Could you check a few things on this drawing? It's one solid part, dimensions in mm from its lowest x, y, z. A direction names the side the tool comes from. Round coordinates to 2 decimals unless told otherwise and drop trailing zeros. Order: outer loops, then holes, each group sorted by start corner. A loop starts at its lowest first (then second) coordinate and runs counter-clockwise, first axis right, second up. Notation, with made-up numbers: (51.5, 49) -> (94.5, 49) arc R24 ccw to (94.5, 81) -> close; hole circle Ø11 at (32.25, -3). An arc over 180 degrees is marked (long way). Use a Markdown table: item, result. Add a question column.
(1) I want a section at C-C, the plane x = 40. Please give me the cut outline in (y, z), then the cut area to 3 significant figures.
(2) I want a section at D-D, the plane y = 83.5. Please give me the cut outline in (x, z), then the cut area to 3 significant figures.
(3) I want a section at B-B, the plane y = 11. Please give me the cut outline in (x, z), then the cut area to 3 significant figures.
(4) I'm going to push flat-ended pins straight in: P1, Ø15, axis at y = 55, z = 23, coming from the -X side; P2, Ø1.5, axis at x = 51, z = 18, coming from the +Y side; P3, Ø8, axis at y = 25, z = 20, coming from the -X side; P4, Ø15, axis at y = 85, z = 23, coming from the +X side. Where does each tip first touch, or does it pass through?
(5) Thinking about a two-plate mould opening in X: for the marked faces 1, 2 and 3, which applies, pulls with the +X half, pulls with the -X half, needs draft (parallel to the pull), parting line crosses it, or undercut?
(6) If I drill on probe 1 along X at (y, z) = (70, 30); probe 2 along X at (y, z) = (78.5, 21.5); probe 3 along Z at (x, y) = (177, 55), over which ranges is the centre line in solid material (lowest first)?
(7) I want a section at A-A, the plane z = 23. Please give me the cut outline in (x, y).
(8) On a 3-axis mill with a long thin cutter (end or side, diameter ignored), from which of +Z, -Z, +X, -X, +Y, -Y can I reach the whole of each face in a straight line? I mean the marked faces 4 and 5. Say none if no direction works.
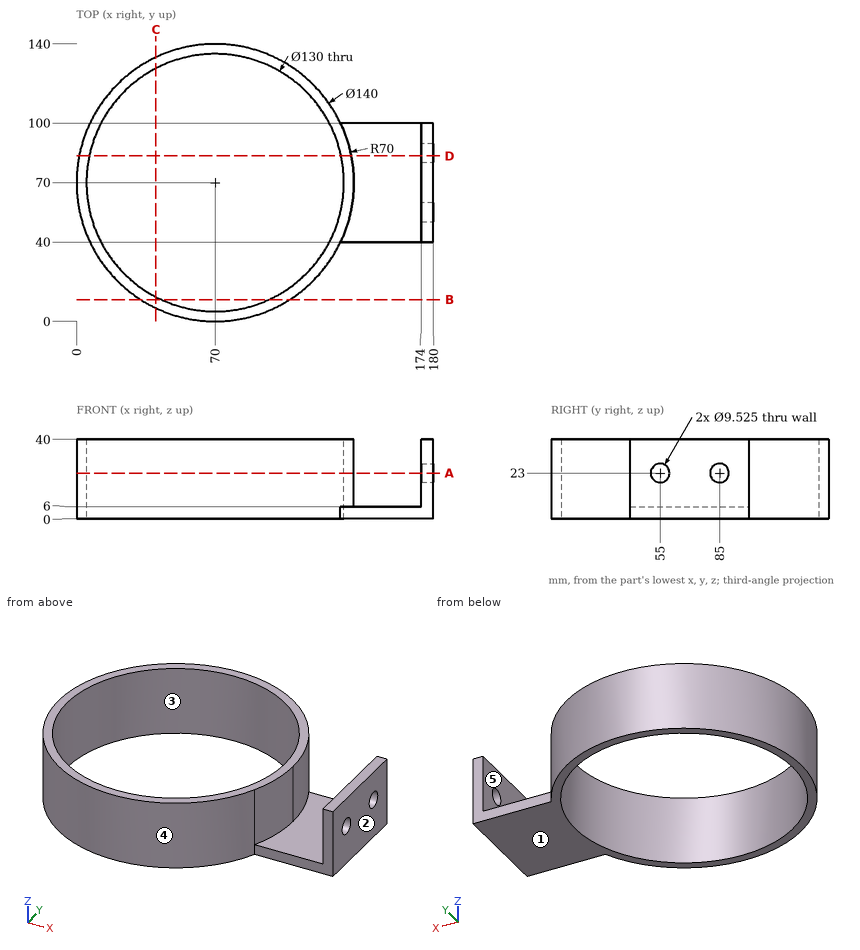
Taken from the geometry:
| question | item | result |
|---|---|---|
| 1 | outline | (6.75, 0) -> (12.34, 0) -> (12.34, 40) -> (6.75, 40) -> close; (127.66, 0) -> (133.25, 0) -> (133.25, 40) -> (127.66, 40) -> close |
| 1 | area | 447 mm2 |
| 2 | outline | (1.31, 0) -> (6.42, 0) -> (6.42, 40) -> (1.31, 40) -> close; (133.58, 0) -> (180, 0) -> (180, 18.48) -> (174, 18.48) -> (174, 6) -> (138.69, 6) -> (138.69, 40) -> (133.58, 40) -> close; (174, 27.52) -> (180, 27.52) -> (180, 40) -> (174, 40) -> close |
| 2 | area | 806 mm2 |
| 3 | outline | (32.33, 0) -> (42.72, 0) -> (42.72, 40) -> (32.33, 40) -> close; (97.28, 0) -> (107.67, 0) -> (107.67, 40) -> (97.28, 40) -> close |
| 3 | area | 831 mm2 |
| 4 | P1 | stops at x = 0.4 |
| 4 | P2 | stops at y = 137.58 |
| 4 | P3 | stops at x = 13.26 |
| 4 | P4 | stops at x = 180 |
| 5 | face 1 | needs draft |
| 5 | face 2 | pulls with the +X half |
| 5 | face 3 | undercut |
| 6 | probe 1 | x = 0 to 5, 135 to 140, 174 to 180 |
| 6 | probe 2 | x = 0.52 to 5.56, 134.44 to 139.48, 174 to 180 |
| 6 | probe 3 | z = 0 to 18.24, 27.76 to 40 |
| 7 | outline | (133.25, 40) arc R70 ccw to (140, 70) arc R70 ccw to (133.25, 100) arc R70 ccw (long way) to start; (174, 40) -> (180, 40) -> (180, 50.24) -> (174, 50.24) -> close; (174, 59.76) -> (180, 59.76) -> (180, 80.24) -> (174, 80.24) -> close; (174, 89.76) -> (180, 89.76) -> (180, 100) -> (174, 100) -> close; hole circle Ø130 at (70, 70) |
| 8 | face 4 | +Z, -Z |
| 8 | face 5 | +Z, +Y, -Y |
